Work out the finished part from the listing and answer in its coordinate system (mm). A direction names the side the tool comes from. Coordinates: 2 decimals unless noted, no trailing zeros. Loops run counter-clockwise (first coordinate to the right, second up) from the corner with the lowest first, then second, coordinate; pieces in that order, holes last. Notation, with made-up numbers: M 78.5,72.25 L 130.5,72.25 A26 cw 130.5,104.25 Z; hole C 59,39.5 d3. An arc over 180 degrees is marked long. Write each question's results on one line, items separated by ' | '.
```python
from build123d import *

# Parameters (mm, degrees)
BOSS_EXTRUDE1_DEPTH    = 9
CUT_EXTRUDE1_DEPTH     = 25
BOSS_EXTRUDE2_DEPTH    = 18
FILLET1_R              = 2
LPATTERN1_COUNT        = 5
LPATTERN1_PITCH        = 6.5
FILLET1_OF_LPATTERN1_R = 2
FILLET2_R              = 8
FILLET3_R              = 5
SKETCH4_R              = 1.5
CUT_EXTRUDE2_DEPTH     = 25
CUT_EXTRUDE3_DEPTH     = 8
SKETCH6_R              = 1.75
BOSS_EXTRUDE3_DEPTH    = 1.5
SKETCH7_R              = 1.75
BOSS_EXTRUDE4_DEPTH    = 1.5
CUT_EXTRUDE4_DEPTH     = 1.5


with BuildPart() as part:
    # Sketch1 → Boss-Extrude1 (new, symmetric)
    with BuildSketch(Plane(origin=(0, 0, 0), x_dir=(0, 0, -1), z_dir=(1, 0, 0))):
        Polygon((78.599259113, -4.792439116), (85.922516335, 2.017105925), (77.751062285, 10.805014591), (71.129492545, 2.15772468), (62.512029777, 2.969258034), (52.963024241, 0), (48.188521473, -1.484629017), (48.188521473, -11.484629017), (58.691485012, -19.145422508), (67.599259113, -47.792439116), (67.599259113, -54.792439116), (78.599259113, -54.792439116), align=None)
        Polygon((62.512029777, 2.969258034), (52.963024241, 0), (32.178218004, 66.843038752), (55.09583129, 73.969258034), align=None)
        with BuildLine():
            Line((85.922516335, 2.017105925), (77.751062285, 10.805014591))
            ThreePointArc((77.751062285, 10.805014591), (86.230743643, 10.496787283), (85.922516335, 2.017105925))
        make_face()
    extrude(amount=BOSS_EXTRUDE1_DEPTH, both=True)

    # Sketch2 → Cut-Extrude1 (cut)
    with BuildSketch(Plane(origin=(9, 0, 0), x_dir=(0, 0, -1), z_dir=(1, 0, 0))):
        Polygon((75.899259113, -47.792439116), (75.899259113, -22.792439116), (63.899259113, -22.792439116), align=None)
    extrude(amount=-CUT_EXTRUDE1_DEPTH, mode=Mode.SUBTRACT)

    # Sketch3 → Boss-Extrude2 (add)
    with BuildSketch(Plane(origin=(9, 0, 0), x_dir=(0, 0, -1), z_dir=(1, 0, 0))):
        Polygon((78.599259113, -47.792439116), (78.599259113, -49.792439116), (82.599259113, -47.792439116), align=None)
        Polygon((78.599259113, -45.792439116), (78.599259113, -47.792439116), (82.599259113, -47.792439116), align=None)
    boss_extrude2 = extrude(amount=-BOSS_EXTRUDE2_DEPTH)

    # Fillet1
    fillet1_edges = [part.edges().sort_by_distance(p)[0] for p in [
        (0, -49.792439116, -78.599259113),
        (0, -45.792439116, -78.599259113),
    ]]
    fillet(fillet1_edges, radius=FILLET1_R)

    # LPattern1: Boss-Extrude2 ×5
    with Locations(*[(0, i * LPATTERN1_PITCH, 0) for i in range(1, LPATTERN1_COUNT)]):
        add(boss_extrude2)

    # Fillet1 of LPattern1
    fillet1_of_lpattern1_edges = [part.edges().sort_by_distance(p)[0] for p in [
        (0, -43.292439116, -78.599259113),
        (0, -39.292439116, -78.599259113),
        (0, -36.792439116, -78.599259113),
        (0, -32.792439116, -78.599259113),
        (0, -30.292439116, -78.599259113),
        (0, -26.292439116, -78.599259113),
        (0, -23.792439116, -78.599259113),
        (0, -19.792439116, -78.599259113),
    ]]
    fillet(fillet1_of_lpattern1_edges, radius=FILLET1_OF_LPATTERN1_R)

    # Fillet2
    # the kernel refuses this fillet: 8 mm, written as the material it takes off along each edge
    with BuildSketch(Plane(origin=(-19.167047595, -11.484629017, -48.188521473), x_dir=(0, -0.5892918069975562, -0.8079202721838058), z_dir=(1, 0, 0))) as fillet2_piece_1:
        with BuildLine():
            CenterArc((FILLET2_R * 0.508352379737, FILLET2_R), FILLET2_R, 216.10676877, 53.89323123)
            Line((-FILLET2_R * 0.299567892447, FILLET2_R * 0.410708193002), (-FILLET2_R * 0.31572629789, FILLET2_R * 0.398922356862))
            Line((-FILLET2_R * 0.31572629789, FILLET2_R * 0.398922356862), (-FILLET2_R * 0.0101670475947, -FILLET2_R * 0.02))
            Line((-FILLET2_R * 0.0101670475947, -FILLET2_R * 0.02), (FILLET2_R * 0.508352379737, -FILLET2_R * 0.02))
            Line((FILLET2_R * 0.508352379737, -FILLET2_R * 0.02), (FILLET2_R * 0.508352379737, 0))
        make_face()
    extrude(amount=38.334095189, mode=Mode.SUBTRACT)
    with BuildSketch(Plane(origin=(-23.590778332, -1.484629017, -48.188521473), x_dir=(0, -1, 0), z_dir=(1, 0, 0))) as fillet2_piece_2:
        with BuildLine():
            CenterArc((5.836311333, 8), FILLET2_R, 203.777574667, 66.222425333)
            Line((-1.484629017, 4.774502768), (-1.631047824, 4.709992823))
            ThreePointArc((-1.631047824, 4.709992823), (-0.895098597, 2.339743255), (-0.152784089, -0.047508129))
            Line((-0.152784089, -0.047508129), (0, -0.16))
            Line((0, -0.16), (5.836311333, -0.16))
            Line((5.836311333, -0.16), (5.836311333, 0))
        make_face()
    extrude(amount=47.181556665, mode=Mode.SUBTRACT)

    # Fillet3
    fillet3_edges = [part.edges().sort_by_distance(p)[0] for p in [
        (0, 66.843038752, -32.178218004),
        (0, 73.969258034, -55.09583129),
    ]]
    fillet(fillet3_edges, radius=FILLET3_R)

    # Sketch4 → Cut-Extrude2 (cut)
    with BuildSketch(Plane(origin=(9, 0, 0), x_dir=(0, 0, -1), z_dir=(1, 0, 0))):
        with Locations((38.437349789, 63.553165001)):
            Circle(SKETCH4_R)
    extrude(amount=-CUT_EXTRUDE2_DEPTH, mode=Mode.SUBTRACT)

    # Sketch5 → Cut-Extrude3 (cut)
    with BuildSketch(Plane(origin=(0, 14.953112663, -48.088564203), x_dir=(1, 0, 0), z_dir=(0, -0.29692580339417163, 0.95490055360688))):
        Polygon((-8, -43.208990891), (8, -43.208990891), (6, -62.708990891), (-6, -62.708990891), align=None)
    extrude(amount=-CUT_EXTRUDE3_DEPTH, mode=Mode.SUBTRACT)

    # Sketch6 → Boss-Extrude3 (add)
    with BuildSketch(Plane(origin=(9, 0, 0), x_dir=(0, 0, -1), z_dir=(1, 0, 0))):
        with Locations((81.83678931, 6.411060258)):
            Circle(SKETCH6_R)
    boss_extrude3 = extrude(amount=BOSS_EXTRUDE3_DEPTH)

    # Sketch7 → Boss-Extrude4 (add)
    with BuildSketch(Plane(origin=(9, 0, 0), x_dir=(0, 0, -1), z_dir=(1, 0, 0))):
        with Locations((56.188521473, -7.417809979)):
            Circle(SKETCH7_R)
    boss_extrude4 = extrude(amount=BOSS_EXTRUDE4_DEPTH)

    # Sketch8 → Cut-Extrude4 (cut)
    with BuildSketch(Plane(origin=(9, 0, 0), x_dir=(0, 0, -1), z_dir=(1, 0, 0))):
        with BuildLine():
            Line((41.354329636, 59.224050938), (49.539044528, 61.769083545))
            ThreePointArc((49.539044528, 61.769083545), (50.809758993, 61.589265105), (51.476316689, 60.492565163))
            Line((51.476316689, 60.492565163), (56.016764829, 17.023958099))
            ThreePointArc((56.016764829, 17.023958099), (54.826962078, 15.398858062), (53.092530542, 16.422736945))
            Line((53.092530542, 16.422736945), (40.367367511, 57.346311403))
            ThreePointArc((40.367367511, 57.346311403), (40.471955982, 58.48958772), (41.354329636, 59.224050938))
        make_face()
    cut_extrude4 = extrude(amount=-CUT_EXTRUDE4_DEPTH, mode=Mode.SUBTRACT)

    # Mirror1: Boss-Extrude3, Boss-Extrude4, Cut-Extrude4 across plane
    add(boss_extrude3.mirror(Plane(origin=(0, 0, 0), x_dir=(0, 0, 1), z_dir=(1, 0, 0))))
    add(boss_extrude4.mirror(Plane(origin=(0, 0, 0), x_dir=(0, 0, 1), z_dir=(1, 0, 0))))
    add(cut_extrude4.mirror(Plane(origin=(0, 0, 0), x_dir=(0, 0, 1), z_dir=(1, 0, 0))), mode=Mode.SUBTRACT)


solid = part.part
```
1) Find section A-A, the plane y = 25.5. Give the vertices of the cut face in (x, z), and give its area (3 significant figures).
Check result:
outline: M -9,-60.16 L 9,-60.16 L 9,-55.13 L 7.5,-55.13 L 7.5,-50.27 L 9,-50.27 L 9,-45.03 L -9,-45.03 L -9,-50.27 L -7.5,-50.27 L -7.5,-55.13 L -9,-55.13 Z | area: 258 mm^2
2) Given pin 1 Ø4 at (x, y) = (-3, -9.5) entering from -Z; pin 2 Ø3 at (x, y) = (-8, 32) entering from +Z; pin 3 Ø7.5 at (x, y) = (4, -52.5) entering from +Z; pin 4 Ø1.8 at (y, z) = (63.55, -38.44) entering from +X, each flat-ended and moving along its own axis, determine where each tip first touches the part or whether it passes through.
Check result:
pin 1: z = -78.6 | pin 2: z = -42.55 | pin 3: z = -67.6 | pin 4: through
3) Which of the six approach directions +Z, -Z, +X, -X, +Y, -Y give full straight-line access (tool end or side, diameter ignored) to faces 1 (the face through (-7.5, 44, -48)), 2 (the face through (0.126, -42.026, -81.132)), 3 (the face through (9.74, 6.937, -83.506))?
Check result:
face 1: -X | face 2: -Z, +X, -X | face 3: +X
4) Find section B-B, the plane y = 44.5. Give the vertices of the cut face in (x, z), and give its area (3 significant figures).
Check result:
outline: M -9,-58.17 L 9,-58.17 L 9,-53.15 L 7.5,-53.15 L 7.5,-44.36 L 9,-44.36 L 9,-39.13 L -9,-39.13 L -9,-44.36 L -7.5,-44.36 L -7.5,-53.15 L -9,-53.15 Z | area: 317 mm^2
5) Straight lines are drawn through the part: probe 1 along Y at (x, z) = (-6, -82); probe 2 along X at (y, z) = (-5.5, -64.5); probe 3 along Z at (x, y) = (3.25, 8). For each, find the intervals that lie inside material, in ascending order. Write a range as [from, to].
Check result:
probe 1: [-48.09, -47.49], [-41.59, -40.99], [-35.09, -34.49], [-28.59, -27.99], [-22.09, -21.49], [-1.63, 12.41] | probe 2: [-9, 9] | probe 3: [-87.62, -75.6], [-61.99, -50.48]
6) For a pull along Y with two mould halves and no side action, classify faces 4 (the face through (9.7, -8.1, -57.8)), 5 (the face through (8.26, 60.48, -45.39)), 6 (the face through (0, -54.792, -73)), 7 (the face through (10.5, 6, -82)) as released by +Y, released by -Y, zero draft, split by the parting line, or undercut.
Check result:
face 4: split by the parting line | face 5: undercut | face 6: released by -Y | face 7: zero draft
